The drawing under review shows one solid part. Ordinate dimensions are in mm from its lowest x, y, z. A direction names the side the tool comes from. Coordinates: 2 decimals unless noted, no trailing zeros. Order: outer loops, then holes, each group sorted by start corner. A loop starts at its lowest first (then second) coordinate and runs counter-clockwise, first axis right, second up. Notation, with made-up numbers: (76.5, 67) -> (103.5, 67) arc R26 cw to (103.5, 85) -> close; hole circle Ø1 at (36.25, -35.5). An arc over 180 degrees is marked (long way). Put each result on its own line as item: value.
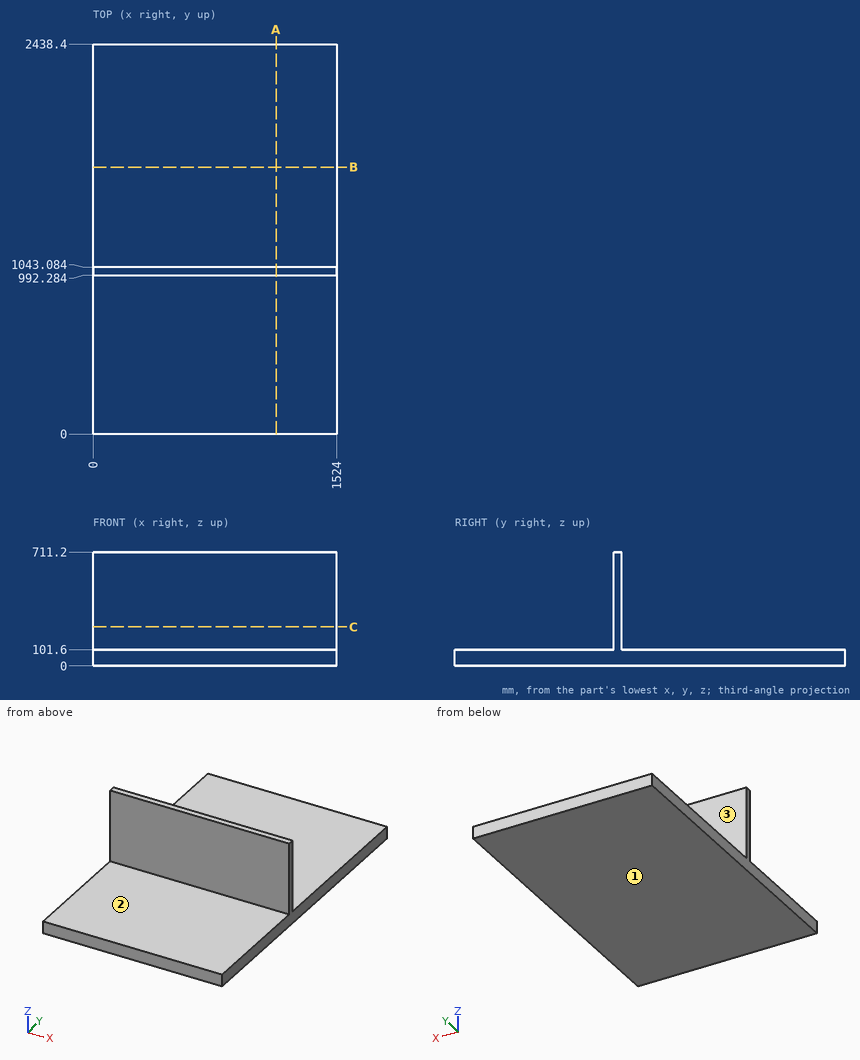
Item 1: For pin 1 Ø6 at (x, z) = (640.5, 387.5) entering from +Y; pin 2 Ø5 at (x, z) = (422, 563) entering from -Y; pin 3 Ø6 at (x, y) = (694, 1715) entering from +Z, all flat-tipped, find the tip position at first contact; note any pin that passes through.
Answers below:
pin 1: y = 1043.08
pin 2: y = 992.28
pin 3: z = 101.6
Item 2: Consider section A-A on x = 1144. Write out the cut boundary in (y, z).
Answers below:
outline: (0, 0) -> (2438.4, 0) -> (2438.4, 101.6) -> (1043.08, 101.6) -> (1043.08, 711.2) -> (992.28, 711.2) -> (992.28, 101.6) -> (0, 101.6) -> close
Item 3: For line 1 (Y direction, x = 312, z = 456.5); line 2 (Z direction, x = 1228, y = 1199.5), list the stretches that pass through material, from the lowest coordinate up. Write a range as from..to.
Answers below:
line 1: 992.28..1043.08
line 2: 0..101.6
Item 4: Consider section C-C on z = 243.5. Write out the cut boundary in (x, y), and give its area (3 significant figures).
Answers below:
outline: (0, 992.28) -> (1524, 992.28) -> (1524, 1043.08) -> (0, 1043.08) -> close
area: 77,400 mm^2
Item 5: Consider section B-B on y = 1668.5. Write out the cut boundary in (x, z), and give its area (3 significant figures).
Answers below:
outline: (0, 0) -> (1524, 0) -> (1524, 101.6) -> (0, 101.6) -> close
area: 155,000 mm^2
Item 6: For the marked faces 1, 2 and 3, list the 3-axis set-ups (+Z, -Z, +X, -X, +Y, -Y) from which the entire face can be reached by the end or side of a thin tool; tool diameter is ignored.
Answers below:
face 1: -Z, +X, -X, +Y, -Y
face 2: +Z, +X, -X, -Y
face 3: +Z, +X, -X, +Y
